For this review, take the finished solid that the model builds, in its own axes (mm). A direction names the side the tool comes from. Coordinates: 2 decimals unless noted, no trailing zeros. Loops run counter-clockwise (first coordinate to the right, second up) from the corner with the lowest first, then second, coordinate; pieces in that order, holes last. Notation, with made-up numbers: (54, -38) -> (83, -38) arc R26 cw to (83, -2) -> close; hole circle Ø1 at (2.25, -13.75). An arc over 180 degrees is marked (long way). Use a Markdown table: item, result.
from build123d import *

# Parameters (mm, degrees)
SKETCH2_R               = 10
BOSS_EXTRUDE1_DEPTH     = 11
SKETCH5_W               = 41
SKETCH5_H               = 10
BOSS_EXTRUDE3_DEPTH     = 37
SKETCH6_R               = 10
CUT_EXTRUDE1_DEPTH      = 1
CUT_EXTRUDE1_DEPTH_BACK = 57


with BuildPart() as part:
    # Sketch2 → Boss-Extrude1 (new body)
    with BuildSketch(Plane(origin=(0, 0, 0), x_dir=(1, 0, 0), z_dir=(0, 1, 0))):
        with BuildLine():
            Line((-46, 0), (-46, 24))
            Line((-46, 24), (-84, 0))
            Line((-84, 0), (-125, 0))
            Line((-125, 0), (-125, 56))
            Line((-125, 56), (-22, 56))
            ThreePointArc((-22, 56), (-6.443650814, 49.556349186), (0, 34))
            Line((0, 34), (0, 0))
            Line((0, 0), (-46, 0))
        make_face()
        with Locations((-22, 34)):
            Circle(SKETCH2_R, mode=Mode.SUBTRACT)
    extrude(amount=BOSS_EXTRUDE1_DEPTH)

    # Sketch5 → Boss-Extrude3 (add)
    with BuildSketch(Plane(origin=(0, 11, 0), x_dir=(1, 0, 0), z_dir=(0, 1, 0))):
        with Locations((-104.5, 51)):
            Rectangle(SKETCH5_W, SKETCH5_H)
        with Locations((-104.5, 5)):
            Rectangle(SKETCH5_W, SKETCH5_H)
    extrude(amount=BOSS_EXTRUDE3_DEPTH)

    # Sketch6 → Cut-Extrude1 (cut, two sides)
    with BuildSketch(Plane.XY) as cut_extrude1_sk:
        with Locations((-104.5, 27)):
            Circle(SKETCH6_R)
    extrude(amount=CUT_EXTRUDE1_DEPTH, mode=Mode.SUBTRACT)
    extrude(cut_extrude1_sk.sketch, amount=-CUT_EXTRUDE1_DEPTH_BACK, mode=Mode.SUBTRACT)


solid = part.part
(1) Take a section at C-C on z = -38.5. Write out the cut boundary in (x, y), plus the area to 3 significant figures.
Found:
| item | result |
|---|---|
| outline | (-125, 0) -> (-30.93, 0) -> (-30.93, 11) -> (-125, 11) -> close; (-13.07, 0) -> (-0.47, 0) -> (-0.47, 11) -> (-13.07, 11) -> close |
| area | 1,170 mm^2 |
(2) Mouldability with a two-part tool opening along Y and no side actions: class faces 5 (the face through (-46, 5, -12)), 6 (the face through (-114.49, 27.44, -4.93)), 7 (the face through (-62, 0, -28)), 8 (the face through (-105, 48, -51)) as pulls with the +Y half, pulls with the -Y half, needs draft (parallel to the pull), parting line crosses it, or undercut.
Found:
| item | result |
|---|---|
| face 5 | needs draft |
| face 6 | undercut |
| face 7 | pulls with the -Y half |
| face 8 | pulls with the +Y half |
(3) For pin 1 Ø1.5 at (x, z) = (-85.5, -23.5) entering from +Y; pin 2 Ø5 at (y, z) = (34.5, -49.5) entering from +X, all flat-tipped, find the tip position at first contact; note any pin that passes through.
Found:
| item | result |
|---|---|
| pin 1 | stops at y = 11 |
| pin 2 | stops at x = -84 |
(4) For faces 1 (the face through (-65, 5, -12)), 2 (the face through (-6.62, 5.42, -49.73)), 3 (the face through (-104.8, 37.5, -10)), 4 (the face through (-84, 29, -5)), list the 3-axis set-ups (+Z, -Z, +X, -X, +Y, -Y) from which the entire face can be reached by the end or side of a thin tool; tool diameter is ignored.
Found:
| item | result |
|---|---|
| face 1 | +Z, +Y, -Y |
| face 2 | -Z, +X, +Y, -Y |
| face 3 | +X, -X, +Y |
| face 4 | +Z, -Z, +X, +Y |
(5) Take a section at B-B on x = -104.5. Write out the cut boundary in (y, z).
Found:
| item | result |
|---|---|
| outline | (0, -56) -> (17, -56) -> (17, -46) -> (11, -46) -> (11, -10) -> (17, -10) -> (17, 0) -> (0, 0) -> close; (37, -56) -> (48, -56) -> (48, -46) -> (37, -46) -> close; (37, -10) -> (48, -10) -> (48, 0) -> (37, 0) -> close |
(6) Take a section at D-D on y = 40. Write out the cut boundary in (x, z).
Found:
| item | result |
|---|---|
| outline | (-125, -56) -> (-84, -56) -> (-84, -46) -> (-125, -46) -> close; (-125, -10) -> (-84, -10) -> (-84, 0) -> (-125, 0) -> close |
(7) For line 1 along Z through (x, y) = (-22, 8.5); line 2 along Y through (x, z) = (-104.5, -6); line 3 along Z through (x, y) = (-101, 13.5), list the stretches that pass through material, from the lowest coordinate up.
Found:
| item | result |
|---|---|
| line 1 | z = -56 to -44, -24 to 0 |
| line 2 | y = 0 to 17, 37 to 48 |
| line 3 | z = -56 to -46, -10 to 0 |
(8) Take a section at A-A on y = 27. Write out the cut boundary in (x, z).
Found:
| item | result |
|---|---|
| outline | (-125, -56) -> (-114.5, -56) -> (-114.5, -46) -> (-125, -46) -> close; (-125, -10) -> (-114.5, -10) -> (-114.5, 0) -> (-125, 0) -> close; (-94.5, -56) -> (-84, -56) -> (-84, -46) -> (-94.5, -46) -> close; (-94.5, -10) -> (-84, -10) -> (-84, 0) -> (-94.5, 0) -> close |
